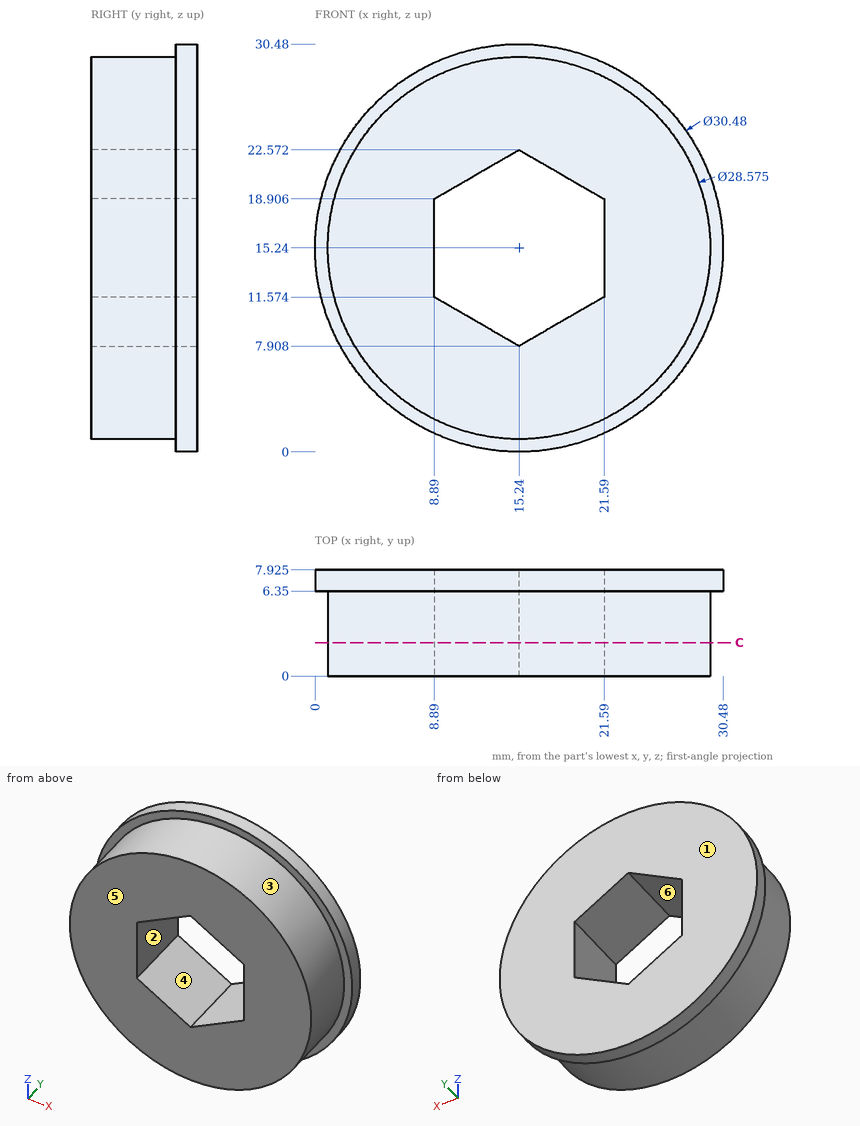
Source: three-view drawing plus pictorial views. Frame: mm from the lowest corner of the part. A direction names the side the tool comes from. Coordinates: 2 decimals unless noted, no trailing zeros. Write each loop counter-clockwise with the first axis right and the second up, starting at its lowest first coordinate (ties: lowest second). Pieces come first, ordered by that corner, then holes. Notation, with made-up numbers: (-20.75, 69) - (11.25, 69) arc R8 cw to (11.25, 80) - close; hole circle Ø1 at (31, 33.25). An arc over 180 degrees is marked (long way). Answer as a JSON object with one key per item and string values.
Q1. Section query C-C, the plane y = 2.5. Output: boundary loops of the cut face in (x, z) (1 decimal), plus the area to 3 significant figures.
Ans:
{"outline": "circle Ø28.6 at (15.2, 15.2); hole (8.9, 11.6) - (15.2, 7.9) - (21.6, 11.6) - (21.6, 18.9) - (15.2, 22.6) - (8.9, 18.9) - close", "area": "502 mm2"}
Q2. First-contact query: pin 1 Ø3.5 at (y, z) = (2, 15.5) entering from +X; pin 2 Ø1 at (x, y) = (24, 4) entering from +Z; pin 3 Ø2 at (y, z) = (2.5, 12.5) entering from -X. Flat tips, straight axial feed; report the tip coordinate or a pass-through.
Ans:
{"pin 1": "stops at x = 29.53", "pin 2": "stops at z = 26.9", "pin 3": "stops at x = 1.06"}
Q3. Set-up query: the marked faces 1 and 2. Return all of +Z, -Z, +X, -X, +Y, -Y with unobstructed straight access to the full face (end or side cutting, diameter ignored); none if empty.
Ans:
{"face 1": "+Z, -Z, +X, -X, +Y", "face 2": "+Y, -Y"}
Q4. Material intervals for line 1 (X direction, y = 1, z = 15.5) (1 decimal); line 2 (X direction, y = 5.75, z = 21) (1 decimal); line 3 (Z direction, x = 20, y = 2.5) (1 decimal), sorted ascending. Write a range as [from, to].
Ans:
{"line 1": "x = [1, 8.9], [21.6, 29.5]", "line 2": "x = [2.2, 12.5], [18, 28.3]", "line 3": "z = [1.8, 10.7], [19.8, 28.7]"}
Q5. Draft query along X for the marked faces 3, 4, 5 and 6. Return one class per face: released by +X, released by -X, zero draft, split by the parting line, or undercut.
Ans:
{"face 3": "split by the parting line", "face 4": "undercut", "face 5": "zero draft", "face 6": "undercut"}
